```python
from build123d import *

# Parameters (mm, degrees)
SKETCH1_W            = 4
SKETCH1_H            = 5
BOSS_EXTRUDE1_DEPTH  = 3.75
SKETCH2_W            = 3.1
SKETCH2_H            = 3.1
CUT_EXTRUDE1_DEPTH   = 5
BOSS_EXTRUDE2_DEPTH  = 7.5
M2_CLEARANCE_HOLE1_D = 2.4
FILLET1_R            = 3.5
FILLET2_R            = 2
FILLET3_R            = 1
SKETCH17_R           = 5
CUT_EXTRUDE2_DEPTH   = 7
SKETCH5_R            = 1.5875
CUT_EXTRUDE3_DEPTH   = 5
FILLET4_R            = 1
SKETCH18_R           = 1.35
CUT_EXTRUDE4_DEPTH   = 5


with BuildPart() as part:
    # Sketch1 → Boss-Extrude1 (new, symmetric)
    with BuildSketch(Plane.XY):
        Rectangle(SKETCH1_W, SKETCH1_H)
    extrude(amount=BOSS_EXTRUDE1_DEPTH, both=True)

    # Sketch2 → Cut-Extrude1 (cut)
    with BuildSketch(Plane(origin=(0, 0, -3.75), x_dir=(-1, 0, 0), z_dir=(0, 0, -1))):
        with Locations((0, -0.55)):
            Rectangle(SKETCH2_W, SKETCH2_H)
    extrude(amount=-CUT_EXTRUDE1_DEPTH, mode=Mode.SUBTRACT)

    # Sketch3 → Boss-Extrude2 (add, symmetric)
    with BuildSketch(Plane(origin=(0, 0, 0), x_dir=(0, 0, -1), z_dir=(1, 0, 0))):
        Polygon((-6.25, 2.5), (3.75, 19.820508076), (11.25, 15.490381057), (3.75, 2.5), align=None)
    extrude(amount=BOSS_EXTRUDE2_DEPTH, both=True)

    # M2 Clearance Hole1 (through all)
    with Locations(Plane.XY.offset(3.75)):
        with Locations((0, -0.5)):
            Hole(M2_CLEARANCE_HOLE1_D / 2)

    # Fillet1
    fillet1_edges = [part.edges().sort_by_distance(p)[0] for p in [
        (-2, 2.5, 0),
        (2, 2.5, 0),
    ]]
    fillet(fillet1_edges, radius=FILLET1_R)

    # Fillet2
    fillet2_edges = [part.edges().sort_by_distance(p)[0] for p in [
        (-7.5, 17.655444566, -7.5),
        (7.5, 17.655444566, -7.5),
        (7.5, 2.5, 1.25),
        (-7.5, 2.5, 1.25),
    ]]
    fillet(fillet2_edges, radius=FILLET2_R - 0.0001)  # a hair under: the kernel refuses the full size

    # Fillet3
    fillet3_edges = [part.edges().sort_by_distance(p)[0] for p in [
        (2, -2.5, 0),
        (-2, -2.5, 0),
    ]]
    fillet(fillet3_edges, radius=FILLET3_R)

    # Sketch17 → Cut-Extrude2 (cut)
    with BuildSketch(Plane(origin=(0, 3.331329387, 5.770031755), x_dir=(1, 0, 0), z_dir=(0, 0.5000000000000039, 0.8660254037844365))):
        with Locations(Location((0, 11.540063509, 0), (0, 0, 270))):
            Circle(SKETCH17_R)
    extrude(amount=-CUT_EXTRUDE2_DEPTH, mode=Mode.SUBTRACT)

    # Sketch5 → Cut-Extrude3 (cut)
    with BuildSketch(Plane(origin=(0, -0.998797632, -1.729968245), x_dir=(-1, 0, 0), z_dir=(0, -0.5000000000000038, -0.8660254037844366))):
        with Locations(Location((0, 11.540063509, 0), (0, 0, 90))):
            Circle(SKETCH5_R)
    extrude(amount=-CUT_EXTRUDE3_DEPTH, mode=Mode.SUBTRACT)

    # Fillet4
    fillet4_edges = [part.edges().sort_by_distance(p)[0] for p in [
        (0, 2.5, 3.75),
    ]]
    fillet(fillet4_edges, radius=FILLET4_R)

    # Sketch18 → Cut-Extrude4 (cut)
    with BuildSketch(Plane(origin=(0, 16.489178689, -9.520031755), x_dir=(1, 0, 0), z_dir=(0, 0.8660254037844366, -0.5000000000000038))):
        with Locations(Location((0, -3.162658774, 0), (0, 0, 270))):
            Circle(SKETCH18_R)
    extrude(amount=-CUT_EXTRUDE4_DEPTH, mode=Mode.SUBTRACT)


solid = part.part
```
Geometry: final body of the model. Coordinates: model frame, mm. A direction names the side the tool comes from. Round coordinates to 2 decimals unless told otherwise and drop trailing zeros. Order: outer loops, then holes, each group sorted by start corner. A loop starts at its lowest first (then second) coordinate and runs counter-clockwise, first axis right, second up. Notation, with made-up numbers: (46, 30) -> (51, 30) arc R21 ccw to (51, 48) -> close; hole circle Ø2 at (54, 20). An arc over 180 degrees is marked (long way). Use one line per item in the form item = value. Start each with the question number.
1. Pin query (flat end, axial travel): pin 1 Ø0.9 at (x, z) = (-0.5, -0.5) entering from +Y; pin 2 Ø3.5 at (x, y) = (-0.5, -1) entering from -Z; pin 3 Ø1 at (x, y) = (-1.5, 14) entering from -Z; pin 4 Ø3 at (y, z) = (17, 1.5) entering from -X. Return the tip coordinate at first contact, or that it passes through.
2. Line query: probe 1 along Y at (x, z) = (-4.5, 4.75); probe 2 along Y at (x, z) = (4, -5); probe 3 along Z at (x, y) = (3, 6.75). Output: solid intervals per line, ascending.
3. Cut plane B-B (y = -0.5). Return the cut outline in (x, z), then the cut area to 3 significant figures.
4. Cut plane D-D (x = 4.5). Return the cut outline in (y, z).
5. Draft query along Y for faces 5 (the face through (-1.32, 16.78, -6.37)), 6 (the face through (0.077, 2.313, 4.167)), 7 (the face through (7.5, 10, -3)). Return one class per face: pulls with the +Y half, pulls with the -Y half, needs draft (parallel to the pull), parting line crosses it, or undercut.
6. Cut plane A-A (x = 0.5). Return the cut outline in (y, z), then the cut area to 3 significant figures.
7. Reachability of faces 1 (the face through (0.07, 7.961, -4.986)), 2 (the face through (-7.5, 10, -3)), 3 (the face through (0, 1, -1)), 4 (the face through (0, 1, 3.75)) from +Z, -Z, +X, -X, +Y, -Y: full face, straight path, thin tool, end or side. Return the list, or none.
Solution:
q1.pin_1 = 7.56
q1.pin_2 = -3.75
q1.pin_3 = -10.68
q1.pin_4 = through
q2.probe_1 = 2.5 to 5.1
q2.probe_2 = 4.67 to 7.99, 13.9 to 19.1
q2.probe_3 = -6.2 to -4.29, -3.39 to 3.8
q3.outline = (-2.04, -3.75) -> (-1.55, -3.75) -> (-1.55, 1.25) -> (-1.2, 1.25) -> (-1.2, 3.75) -> (-2.04, 3.75) -> close; (1.2, 1.25) -> (1.55, 1.25) -> (1.55, -3.75) -> (2.04, -3.75) -> (2.04, 3.75) -> (1.2, 3.75) -> close
q3.area = 9.04 mm^2
q4.outline = (2.35, -3.75) -> (2.5, -3.75) -> (15.49, -11.25) -> (19.82, -3.75) -> (15.21, -1.09) -> (11.71, -7.15) -> (7.94, -4.97) -> (11.44, 1.09) -> (2.5, 6.25) -> (2.5, 4.75) arc R1 cw to (2.35, 4.23) -> close
q5.face_5 = undercut
q5.face_6 = pulls with the -Y half
q5.face_7 = needs draft
q6.outline = (-2.5, -3.75) -> (-2.1, -3.75) -> (-2.1, 1.25) -> (-1.59, 1.25) -> (-1.59, 3.75) -> (-2.5, 3.75) -> close; (0.59, 1.25) -> (1, 1.25) -> (1, -3.75) -> (2.5, -3.75) -> (7.69, -6.75) -> (8.52, -5.31) -> (5.52, -3.57) -> (9.02, 2.49) -> (2.5, 6.25) -> (2.5, 4.75) arc R1 cw to (1.5, 3.75) -> (0.59, 3.75) -> close; (10.3, -8.25) -> (15.49, -11.25) -> (17.44, -7.87) -> (15.26, -6.6) -> (14.13, -8.55) -> (11.13, -6.82) -> close; (16.51, -4.43) -> (18.7, -5.7) -> (19.82, -3.75) -> (17.63, -2.49) -> close
q6.area = 87.3 mm^2
q7.face_1 = none
q7.face_2 = +Z, -Z, -X, +Y, -Y
q7.face_3 = -Z
q7.face_4 = +Z, +X, -X, -Y
